Could you check a few things on this model? Use its own coordinates, in mm. A direction names the side the tool comes from. Give positions to 0.01 mm unless a question says otherwise; leave off trailing zeros. Order: outer loops, then holes, each group sorted by start corner. A loop starts at its lowest first (then second) coordinate and runs counter-clockwise, first axis right, second up. Notation, with made-up numbers: (34.25, 60.5) - (85.25, 60.5) arc R23 ccw to (85.25, 76.5) - close; hole circle Ø2 at (17.5, -18.75). An arc over 180 degrees is marked (long way). One line per question, with ' | ' between items. Start each with the question number.
1. Imagine slicing it at C-C (y = 35.5). Please give me the cut outline in (x, z).
2. I need wall thicknesses on probe 1 along Y at (x, z) = (82.5, 2.7); probe 2 along X at (y, z) = (31, 1.25); probe 3 along Y at (x, z) = (43.5, -13.5). Which ranges of each line are inside material? Lowest first, please. Write a range as from..to.
3. Imagine slicing it at A-A (y = 14.5). Please give me the cut outline in (x, z).
4. Imagine slicing it at D-D (x = 82.5). Please give me the cut outline in (y, z).
5. Which directions (+Z, -Z, +X, -X, +Y, -Y) give clear straight access to the entire face, cutting with the end or side of a thin tool? Please do faces 5 (the cylindrical face through (45.65, -2.93, -0.6)), 6 (the flat face through (80.75, 37, 2)), 7 (the cylindrical face through (-4.859, -4.797, -6.26)).
6. If we mould it in two halves opening along X, with no side actions, what happens to faces 1 (the flat face through (96, 20, -6)), 2 (the flat face through (45, 45, -16.4)), 3 (the cylindrical face through (6.763, 5.176, 1.775)), 4 (the flat face through (-6, 20, -6))? For each: released by +X, released by -X, zero draft, split by the parting line, or undercut.
7. For P1, Ø6, axis at x = 82, y = 2.5, coming from the -Z side, with a flat end and sliding along its axis, tell me the tip position at first contact or that it passes through.
8. Imagine slicing it at B-B (x = 13.5). Please give me the cut outline in (y, z), and give its area (3 significant figures).
```python
from build123d import *

# Parameters (mm, degrees)
ESQUISSE1_W                     = 102
ESQUISSE1_H                     = 52
ESQUISSE1_W_2                   = 90
ESQUISSE1_H_2                   = 40
EXTRU_MINCE1_DEPTH              = 3.6
ESQUISSE2_W                     = 9.25
ESQUISSE2_H                     = 40
BOSS_EXTRU_1_DEPTH              = 3.6
ESQUISSE3_R                     = 1
ESQUISSE3_W                     = 4.29767414
ESQUISSE3_H                     = 26.5
ENL_V_MAT_EXTRU_1_DEPTH         = 3.6
ESQUISSE5_W                     = 102
ESQUISSE5_H                     = 52
ESQUISSE5_W_2                   = 97
ESQUISSE5_H_2                   = 47
EXTRU_MINCE2_DEPTH              = 20
CONG_1_R                        = 4
CONG_2_R                        = 2
ENL_V_DE_MAT_EXTRU_MINCE1_DEPTH = 2


with BuildPart() as part:
    # Esquisse1 → Extru.-Mince1 (new body)
    with BuildSketch(Plane.XY):
        with Locations((45, 20)):
            Rectangle(ESQUISSE1_W, ESQUISSE1_H)
        with Locations((45, 20)):
            Rectangle(ESQUISSE1_W_2, ESQUISSE1_H_2, mode=Mode.SUBTRACT)
    extrude(amount=EXTRU_MINCE1_DEPTH)

    # Esquisse2 → Boss.-Extru.1 (add)
    with BuildSketch(Plane.XY):
        with Locations((4.625, 20)):
            Rectangle(ESQUISSE2_W, ESQUISSE2_H)
        Polygon((90, 40), (90, 0), (80.75, 0), (80.75, 6.5), (85, 6.5), (85, 33.5), (80.75, 33.5), (80.75, 40), align=None)
    extrude(amount=BOSS_EXTRU_1_DEPTH)

    # Esquisse3 → Enlèv. mat.-Extru.1 (cut)
    with BuildSketch(Plane.XY):
        with Locations((7.5, 35.5)):
            Circle(ESQUISSE3_R)
        with Locations((7.5, 4.5)):
            Circle(ESQUISSE3_R)
        with Locations((82.5, 35.5)):
            Circle(ESQUISSE3_R)
        with Locations((82.5, 4.5)):
            Circle(ESQUISSE3_R)
        with Locations((10.39883707, 20)):
            Rectangle(ESQUISSE3_W, ESQUISSE3_H)
    extrude(amount=ENL_V_MAT_EXTRU_1_DEPTH, mode=Mode.SUBTRACT)

    # Esquisse5 → Extru.-Mince2 (add)
    with BuildSketch(Plane.XY.offset(3.6)):
        with Locations((45, 20)):
            Rectangle(ESQUISSE5_W, ESQUISSE5_H)
        with Locations((45, 20)):
            Rectangle(ESQUISSE5_W_2, ESQUISSE5_H_2, mode=Mode.SUBTRACT)
    extrude(amount=-EXTRU_MINCE2_DEPTH)

    # Congé1
    cong_1_edges = [part.edges().sort_by_distance(p)[0] for p in [
        (-6, 46, -6.4),
        (96, 46, -6.4),
        (96, -6, -6.4),
        (-6, -6, -6.4),
    ]]
    fillet(cong_1_edges, radius=CONG_1_R)

    # Congé2
    cong_2_edges = [part.edges().sort_by_distance(p)[0] for p in [
        (45, -3.5, 0),
        (93.5, 20, 0),
        (93.5, -3.5, -8.2),
        (-3.5, -3.5, -8.2),
        (-3.5, 43.5, -8.2),
        (93.5, 43.5, -8.2),
        (45, 43.5, 0),
        (-3.5, 20, 0),
    ]]
    fillet(cong_2_edges, radius=CONG_2_R)

    # Esquisse6 → Enlèv. de mat.-Extru.-Mince1 (cut)
    with BuildSketch(Plane(origin=(0, 0, -16.4), x_dir=(-1, 0, 0), z_dir=(0, 0, -1))):
        with BuildLine():
            Line((1.5, 44.5), (-91.5, 44.5))
            ThreePointArc((-91.5, 44.5), (-93.621320344, 43.621320344), (-94.5, 41.5))
            Line((-94.5, 41.5), (-94.5, -1.5))
            ThreePointArc((-94.5, -1.5), (-93.621320344, -3.621320344), (-91.5, -4.5))
            Line((-91.5, -4.5), (1.5, -4.5))
            ThreePointArc((1.5, -4.5), (3.621320344, -3.621320344), (4.5, -1.5))
            Line((4.5, -1.5), (4.5, 41.5))
            ThreePointArc((4.5, 41.5), (3.621320344, 43.621320344), (1.5, 44.5))
        make_face()
        with BuildLine():
            Line((1.5, 43.5), (-91.5, 43.5))
            ThreePointArc((-91.5, 43.5), (-92.914213562, 42.914213562), (-93.5, 41.5))
            Line((-93.5, 41.5), (-93.5, -1.5))
            ThreePointArc((-93.5, -1.5), (-92.914213562, -2.914213562), (-91.5, -3.5))
            Line((-91.5, -3.5), (1.5, -3.5))
            ThreePointArc((1.5, -3.5), (2.914213562, -2.914213562), (3.5, -1.5))
            Line((3.5, -1.5), (3.5, 41.5))
            ThreePointArc((3.5, 41.5), (2.914213562, 42.914213562), (1.5, 43.5))
        make_face(mode=Mode.SUBTRACT)
    extrude(amount=-ENL_V_DE_MAT_EXTRU_MINCE1_DEPTH, mode=Mode.SUBTRACT)


solid = part.part
```
Results found:
1) outline: (-6, -16.4) - (-4.5, -16.4) - (-4.5, -14.4) - (-3.5, -14.4) - (-3.5, -2) arc R2 cw to (-1.5, 0) - (6.5, 0) - (6.5, 3.6) - (-6, 3.6) - close; (8.5, 0) - (9.25, 0) - (9.25, 3.6) - (8.5, 3.6) - close; (80.75, 0) - (81.5, 0) - (81.5, 3.6) - (80.75, 3.6) - close; (83.5, 0) - (91.5, 0) arc R2 cw to (93.5, -2) - (93.5, -14.4) - (94.5, -14.4) - (94.5, -16.4) - (96, -16.4) - (96, 3.6) - (83.5, 3.6) - close
2) probe 1: y = -6..3.5, 5.5..6.5, 33.5..34.5, 36.5..46 | probe 2: x = -6..8.25, 85..96 | probe 3: y = -6..-3.5, 43.5..46
3) outline: (-6, -16.4) - (-4.5, -16.4) - (-4.5, -14.4) - (-3.5, -14.4) - (-3.5, -2) arc R2 cw to (-1.5, 0) - (8.25, 0) - (8.25, 3.6) - (-6, 3.6) - close; (85, 0) - (91.5, 0) arc R2 cw to (93.5, -2) - (93.5, -14.4) - (94.5, -14.4) - (94.5, -16.4) - (96, -16.4) - (96, 3.6) - (85, 3.6) - close
4) outline: (-6, -16.4) - (-4.5, -16.4) - (-4.5, -14.4) - (-3.5, -14.4) - (-3.5, -2) arc R2 cw to (-1.5, 0) - (3.5, 0) - (3.5, 3.6) - (-6, 3.6) - close; (5.5, 0) - (6.5, 0) - (6.5, 3.6) - (5.5, 3.6) - close; (33.5, 0) - (34.5, 0) - (34.5, 3.6) - (33.5, 3.6) - close; (36.5, 0) - (41.5, 0) arc R2 cw to (43.5, -2) - (43.5, -14.4) - (44.5, -14.4) - (44.5, -16.4) - (46, -16.4) - (46, 3.6) - (36.5, 3.6) - close
5) face 5: -Z | face 6: +Z, -Z | face 7: +Z, -Z, -X, -Y
6) face 1: released by +X | face 2: zero draft | face 3: undercut | face 4: released by -X
7) P1: stops at z = 0
8) outline: (-6, -16.4) - (-4.5, -16.4) - (-4.5, -14.4) - (-3.5, -14.4) - (-3.5, -2) arc R2 cw to (-1.5, 0) - (0, 0) - (0, 3.6) - (-6, 3.6) - close; (40, 0) - (41.5, 0) arc R2 cw to (43.5, -2) - (43.5, -14.4) - (44.5, -14.4) - (44.5, -16.4) - (46, -16.4) - (46, 3.6) - (40, 3.6) - close | area: 123 mm2
